Input: part model. Units: mm. Frame: model coordinates. Round coordinates to 2 decimals unless told otherwise and drop trailing zeros. Loops run counter-clockwise (first coordinate to the right, second up) from the corner with the lowest first, then second, coordinate; pieces in that order, holes last. Notation, with made-up numbers: (-2, -28.5) - (47, -28.5) arc R9 ccw to (47, -18.5) - close; hole circle Ø8 at (10, -9.5). An arc over 180 degrees is marked (long way). One line per question, with ' | ' between items. Start each with the question number.
Item 1: Section C-C, the plane x = 7.5. Return loops of the section in (y, z), plus the area to 3 significant figures.
Item 2: Section A-A, the plane x = 0. Return loops of the section in (y, z) (3 decimals), plus the area to 3 significant figures.
Item 3: Section D-D, the plane z = 3.3. Return loops of the section in (x, y) (3 decimals).
Item 4: Section B-B, the plane y = 0. Return loops of the section in (x, z) (3 decimals), plus the area to 3 significant figures.
Item 5: Material intervals for line 1 along X through (y, z) = (0.5, 3.4); line 2 along Y through (x, z) = (8, 4.6); line 3 along X through (y, z) = (1.5, 4.75), sorted ascending.
Item 6: First-contact query: pin 1 (1.5 mm diameter, centred on x = 12.5, z = 3.5, fed in from -Y); pin 2 (5.5 mm diameter, centred on x = -6.6, y = -11.44, fed in from -Z); pin 3 (2 mm diameter, centred on y = 5, z = 1.5, fed in from +X). Flat tips, straight axial feed; report the tip coordinate or a pass-through.
Item 7: Draft query along X for faces 1 (the face through (14.599, 1.066, 2.576)), 2 (the face through (15.748, 4.959, 2.504)), 3 (the face through (-0.2, -3.4, 5.08)). Return one class per face: pulls with the +X half, pulls with the -X half, needs draft (parallel to the pull), parting line crosses it, or undercut.
```python
from build123d import *

# Parameters (mm, degrees)
SKETCH1_R           = 16.51
BOSS_EXTRUDE1_DEPTH = 5.08
SKETCH2_R           = 3.175
CUT_EXTRUDE1_DEPTH  = 5.08
SKETCH3_R           = 1.7526
CUT_EXTRUDE2_DEPTH  = 5.08
CIRPATTERN1_COUNT   = 6


with BuildPart() as part:
    # Sketch1 → Boss-Extrude1 (new body)
    with BuildSketch(Plane.XY):
        Circle(SKETCH1_R)
    extrude(amount=BOSS_EXTRUDE1_DEPTH)

    # Sketch2 → Cut-Extrude1 (cut)
    with BuildSketch(Plane.XY.offset(5.08)):
        Circle(SKETCH2_R)
    extrude(amount=-CUT_EXTRUDE1_DEPTH, mode=Mode.SUBTRACT)

    # Sketch3 → Cut-Extrude2 (cut)
    with BuildSketch(Plane.XY.offset(5.08)):
        with Locations((-13.208, 0)):
            Circle(SKETCH3_R)
    cut_extrude2 = extrude(amount=-CUT_EXTRUDE2_DEPTH, mode=Mode.SUBTRACT)

    # CirPattern1: Cut-Extrude2 ×6 about axis
    cirpattern1_axis = Axis((0, 0, 0), (0, 0, 1))
    for i in range(1, CIRPATTERN1_COUNT):
        add(cut_extrude2.rotate(cirpattern1_axis, i * 360 / CIRPATTERN1_COUNT), mode=Mode.SUBTRACT)


solid = part.part
```
Return value:
1) outline: (-14.71, 0) - (-12.94, 0) - (-12.94, 5.08) - (-14.71, 5.08) - close; (-9.93, 0) - (9.93, 0) - (9.93, 5.08) - (-9.93, 5.08) - close; (12.94, 0) - (14.71, 0) - (14.71, 5.08) - (12.94, 5.08) - close | area: 119 mm2
2) outline: (-16.51, 0) - (-3.175, 0) - (-3.175, 5.08) - (-16.51, 5.08) - close; (3.175, 0) - (16.51, 0) - (16.51, 5.08) - (3.175, 5.08) - close | area: 135 mm2
3) outline: circle Ø33.02 at (0, 0); hole circle Ø3.505 at (-13.208, 0); hole circle Ø3.505 at (-6.604, -11.438); hole circle Ø3.505 at (-6.604, 11.438); hole circle Ø6.35 at (0, 0); hole circle Ø3.505 at (6.604, -11.438); hole circle Ø3.505 at (6.604, 11.438); hole circle Ø3.505 at (13.208, 0)
4) outline: (-16.51, 0) - (-14.961, 0) - (-14.961, 5.08) - (-16.51, 5.08) - close; (-11.455, 0) - (-3.175, 0) - (-3.175, 5.08) - (-11.455, 5.08) - close; (3.175, 0) - (11.455, 0) - (11.455, 5.08) - (3.175, 5.08) - close; (14.961, 0) - (16.51, 0) - (16.51, 5.08) - (14.961, 5.08) - close | area: 99.9 mm2
5) line 1: -16.5 to -14.89, -11.53 to -3.14, 3.14 to 11.53, 14.89 to 16.5 | line 2: -14.44 to -12.5, -10.38 to 10.38, 12.5 to 14.44 | line 3: -16.44 to -14.11, -12.3 to -2.8, 2.8 to 12.3, 14.11 to 16.44
6) pin 1: y = -11.6 | pin 2: z = 0 | pin 3: x = 16.02
7) face 1: undercut | face 2: parting line crosses it | face 3: needs draft
